from build123d import *

# Parameters (mm, degrees)
SKETCH3_W            = 57.15
SKETCH3_H            = 72
BOSS_EXTRUDE1_DEPTH  = 5
SKETCH5_R            = 5
SKETCH5_R_2          = 3.025
BOSS_EXTRUDE2_DEPTH  = 0.5
CUT_EXTRUDE1_START   = -4.5
SKETCH6_R            = 3.025
CUT_EXTRUDE1_DEPTH   = 4.5
SKETCH8_W            = 9.600002072
SKETCH8_H            = 47.399999581
CUT_EXTRUDE2_DEPTH   = 2
SKETCH10_W           = 57.15
SKETCH10_H           = 2
BOSS_EXTRUDE3_DEPTH  = 15
SKETCH11_W           = 5.5
SKETCH11_H           = 11
BOSS_EXTRUDE4_DEPTH  = 5
M4_CLEARANCE_HOLE1_D = 4.8
FILLET2_R            = 3


with BuildPart() as part:
    # Sketch3 → Boss-Extrude1 (new body)
    with BuildSketch(Plane.XY):
        Rectangle(SKETCH3_W, SKETCH3_H)
    extrude(amount=BOSS_EXTRUDE1_DEPTH)

    # Sketch5 → Boss-Extrude2 (add)
    # profile 1 of 4: a face of its own
    with BuildSketch(Plane.XY.offset(5)):
        with Locations((17.621, 28.575)):
            Circle(SKETCH5_R)
        with Locations((17.621, 28.575)):
            Circle(SKETCH5_R_2, mode=Mode.SUBTRACT)
    # profile 2 of 4: a face of its own
    with BuildSketch(Plane.XY.offset(5)):
        with Locations((17.621, -28.575)):
            Circle(SKETCH5_R)
        with Locations((17.621, -28.575)):
            Circle(SKETCH5_R_2, mode=Mode.SUBTRACT)
    # profile 3 of 4: a face of its own
    with BuildSketch(Plane.XY.offset(5)):
        with Locations((-1.429, -28.575)):
            Circle(SKETCH5_R)
        with Locations((-1.429, -28.575)):
            Circle(SKETCH5_R_2, mode=Mode.SUBTRACT)
    # profile 4 of 4: a face of its own
    with BuildSketch(Plane.XY.offset(5)):
        with Locations((-1.429, 28.575)):
            Circle(SKETCH5_R)
        with Locations((-1.429, 28.575)):
            Circle(SKETCH5_R_2, mode=Mode.SUBTRACT)
    extrude(amount=BOSS_EXTRUDE2_DEPTH)

    # Sketch6 → Cut-Extrude1 (cut)
    with BuildSketch(Plane.XY.offset(5).offset(CUT_EXTRUDE1_START)):
        with Locations((-1.429, 28.575)):
            Circle(SKETCH6_R)
        with Locations((17.621, 28.575)):
            Circle(SKETCH6_R)
        with Locations((-1.429, -28.575)):
            Circle(SKETCH6_R)
        with Locations((17.621, -28.575)):
            Circle(SKETCH6_R)
    extrude(amount=CUT_EXTRUDE1_DEPTH, mode=Mode.SUBTRACT)

    # Sketch8 → Cut-Extrude2 (cut)
    with BuildSketch(Plane.XY.offset(5)):
        with Locations((-0.315001587, -0.172003205)):
            Rectangle(SKETCH8_W, SKETCH8_H)
        Polygon((15.508001492, 19.203997676), (27.508001492, 19.203997676), (27.508001492, -18.696002324), (15.508003148, -18.696002324), align=None)
    extrude(amount=-CUT_EXTRUDE2_DEPTH, mode=Mode.SUBTRACT)

    # Sketch10 → Boss-Extrude3 (add)
    with BuildSketch(Plane.XY.offset(5)):
        with Locations((0, 35)):
            Rectangle(SKETCH10_W, SKETCH10_H)
        with Locations((0, -35)):
            Rectangle(SKETCH10_W, SKETCH10_H)
    extrude(amount=BOSS_EXTRUDE3_DEPTH)

    # Sketch11 → Boss-Extrude4 (add)
    with BuildSketch(Plane(origin=(0, 0, 0), x_dir=(-1, 0, 0), z_dir=(0, 0, -1))):
        with Locations((-13.825, 41.5)):
            Rectangle(SKETCH11_W, SKETCH11_H)
        with Locations((-8.325, 41.5)):
            Rectangle(SKETCH11_W, SKETCH11_H)
    boss_extrude4 = extrude(amount=-BOSS_EXTRUDE4_DEPTH)

    # M4 Clearance Hole1 (through all)
    with Locations(Plane.XY.offset(5)):
        with Locations((11.075, 41.5)):
            m4_clearance_hole1 = Hole(M4_CLEARANCE_HOLE1_D / 2)

    # Mirror1: Boss-Extrude4, M4 Clearance Hole1 across plane
    add(boss_extrude4.mirror(Plane.ZX))
    add(m4_clearance_hole1.mirror(Plane.ZX), mode=Mode.SUBTRACT)

    # Fillet2
    fillet2_edges = [part.edges().sort_by_distance(p)[0] for p in [
        (5.575, 36, 2.5),
        (16.575, 36, 2.5),
        (16.575, 47, 2.5),
        (5.575, 47, 2.5),
        (16.575, -36, 2.5),
        (5.575, -36, 2.5),
        (5.575, -47, 2.5),
        (16.575, -47, 2.5),
    ]]
    fillet(fillet2_edges, radius=FILLET2_R)


solid = part.part
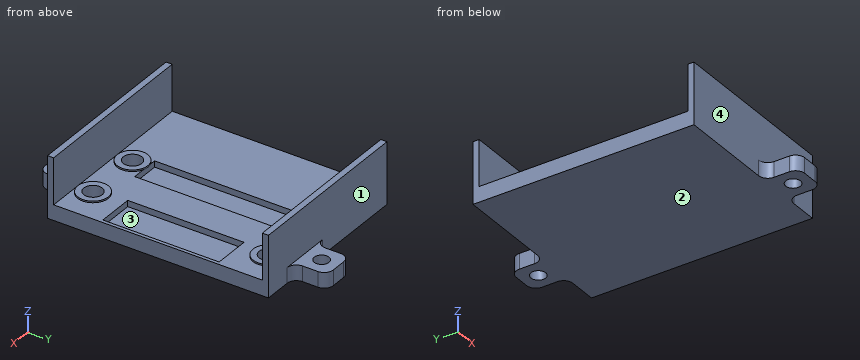
The model under review builds one solid part; all positions refer to its coordinate system, in mm. Face numbers are marked on the shaded views. Round coordinates to 2 decimals unless told otherwise and drop trailing zeros. Loops run counter-clockwise (first coordinate to the right, second up) from the corner with the lowest first, then second, coordinate; pieces in that order, holes last. Notation, with made-up numbers: (7.5, 49.25) -> (21.5, 49.25) arc R16 cw to (21.5, 68.25) -> close; hole circle Ø11 at (72, 64.5). An arc over 180 degrees is marked (long way). One line per question, with ' | ' between items. Start each with the question number.
Item 1: Add section B-B, the plane z = 17.25. Write out the cut boundary in (x, y) (3 decimals), then the cut area to 3 significant figures.
Item 2: Draft analysis for pull direction Y (two halves, no side actions). For the marked faces 1, 2, 3 and 4, state which applies: +Y half, -Y half, draft (parallel to the pull), parting line (faces both ways), or undercut.
Item 3: Wall thickness on line 1 along Y through (x, z) = (14, 11.25); line 2 along Z through (x, y) = (12, -31); line 3 along Y through (x, z) = (11.5, 1.75): over which ranges is each line inside the solid? List them lowest first. Write a range as [from, to].
Item 4: Add section C-C, the plane x = -21. Write out the cut boundary in (y, z), then the cut area to 3 significant figures.
Item 5: For pin 1 (4 mm diameter, centred on y = -42.5, z = 3, fed in from +X) (3 decimals); pin 2 (3 mm diameter, centred on x = -2.5, z = 15, fed in from +Y); pin 3 (1.6 mm diameter, centred on x = 0, z = 4, fed in from -Y); pin 4 (8 mm diameter, centred on x = 21, y = -17.5, fed in from -Z), all flat-tipped, find the tip position at first contact; note any pin that passes through.
Item 6: Add section A-A, the plane y = 41.5. Write out the cut boundary in (x, z) (3 decimals).
Return value:
1) outline: (-28.575, -36) -> (28.575, -36) -> (28.575, -34) -> (-28.575, -34) -> close; (-28.575, 34) -> (28.575, 34) -> (28.575, 36) -> (-28.575, 36) -> close | area: 229 mm2
2) face 1: +Y half | face 2: draft | face 3: undercut | face 4: -Y half
3) line 1: y = [-36, -34], [34, 36] | line 2: z = [0, 5] | line 3: y = [-47, -43.86], [-39.14, 39.14], [43.86, 47]
4) outline: (-36, 0) -> (36, 0) -> (36, 20) -> (34, 20) -> (34, 5) -> (-34, 5) -> (-34, 20) -> (-36, 20) -> close | area: 420 mm2
5) pin 1: stops at x = 16.575 | pin 2: stops at y = 36 | pin 3: stops at y = -36 | pin 4: stops at z = 0
6) outline: (5.575, 0) -> (8.675, 0) -> (8.675, 5) -> (5.575, 5) -> close; (13.475, 0) -> (16.575, 0) -> (16.575, 5) -> (13.475, 5) -> close
